For this review, take the finished solid that the model builds, in its own axes (mm). Coordinates: 2 decimals unless noted, no trailing zeros. Loops run counter-clockwise (first coordinate to the right, second up) from the corner with the lowest first, then second, coordinate; pieces in that order, holes last. Notation, with made-up numbers: (57.25, -9) -> (79.25, -9) arc R21 ccw to (79.25, 14) -> close; hole circle Ø3 at (49, 10.5). An arc over 180 degrees is marked (long way). Use a Markdown table: item, result.
from build123d import *

# Parameters (mm, degrees)
F0_R     = 2.0193
F1_DEPTH = 3.175


with BuildPart() as f1:
    # F0 (on Front) → F1 (new body)
    with BuildSketch(Plane.XZ):
        Polygon((-80.645, -94.45625), (59.055, -94.45625), (59.055, 122.2375), (33.655, 122.2375), (-80.645, -18.25625), align=None)
        with Locations((-74.295, -62.70625)):
            Circle(F0_R, mode=Mode.SUBTRACT)
        with Locations((-74.295, -24.60625)):
            Circle(F0_R, mode=Mode.SUBTRACT)
        with Locations((52.705, -62.70625)):
            Circle(F0_R, mode=Mode.SUBTRACT)
        with Locations((52.705, 16.66875)):
            Circle(F0_R, mode=Mode.SUBTRACT)
        with Locations((52.705, 96.04375)):
            Circle(F0_R, mode=Mode.SUBTRACT)
    extrude(amount=F1_DEPTH)


solid = f1.part
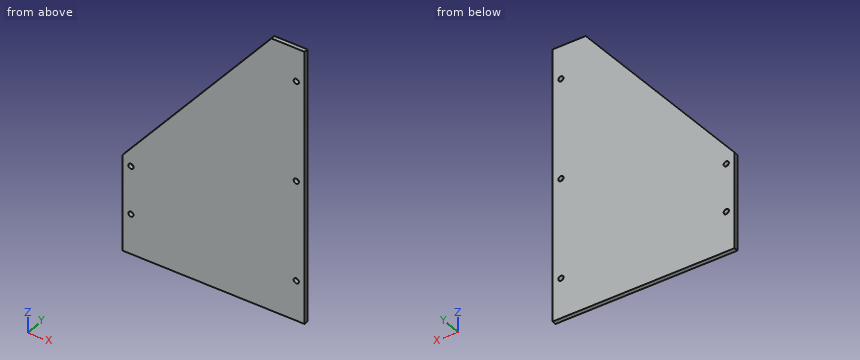
(1) Take a section at B-B on z = 9.5. Write out the cut boundary in (x, y) (3 decimals), plus the area to 3 significant figures.
Found:
| item | result |
|---|---|
| outline | (-58.064, -3.175) -> (59.055, -3.175) -> (59.055, 0) -> (-58.064, 0) -> close |
| area | 372 mm^2 |
(2) Take a section at A-A on y = -2. Write out the cut boundary in (x, z) (1 decimal).
Found:
| item | result |
|---|---|
| outline | (-80.6, -94.5) -> (59.1, -94.5) -> (59.1, 122.2) -> (33.7, 122.2) -> (-80.6, -18.3) -> close; hole circle Ø4 at (-74.3, -62.7); hole circle Ø4 at (-74.3, -24.6); hole circle Ø4 at (52.7, -62.7); hole circle Ø4 at (52.7, 16.7); hole circle Ø4 at (52.7, 96) |
(3) Take a section at C-C on x = 31. Write out the cut boundary in (y, z) (3 decimals).
Found:
| item | result |
|---|---|
| outline | (-3.175, -94.456) -> (0, -94.456) -> (0, 118.974) -> (-3.175, 118.974) -> close |
(4) For line 1 along X through (y, z) = (-1.7, 94.5) (3 decimals); line 2 along X through (y, z) = (-0.2, 30.5) (3 decimals); line 3 along Z through (x, y) = (19, -2.9), list the stretches that pass through material, from the lowest coordinate up.
Found:
| item | result |
|---|---|
| line 1 | x = 11.089 to 51.403, 54.007 to 59.055 |
| line 2 | x = -40.979 to 59.055 |
| line 3 | z = -94.46 to 104.22 |
